```python
from build123d import *

# Parameters (mm, degrees)
F0_R     = 2.5
F1_DEPTH = 5
F2_R     = 15
F2_R_2   = 2.5
F3_DEPTH = 100
F4_SIZE2 = 99.99999
F4_SIZE  = 4.99999


# Not quite as in the source:
# - a fillet or chamfer is up to 0.001 mm smaller than in the source, because OpenCascade refuses the exact size


with BuildPart() as f1:
    # F0 (on Top) → F1 (new body)
    with BuildSketch(Plane.XY):
        with BuildLine():
            Line((7.4939975981, -22.8), (14.0512454964, -5.25))
            ThreePointArc((14.0512454964, -5.25), (0, 15), (-14.0512454964, -5.25))
            Line((-14.0512454964, -5.25), (-7.4939975981, -22.8))
            ThreePointArc((-7.4939975981, -22.8), (0, -28), (7.4939975981, -22.8))
        make_face()
        with Locations((0, -20)):
            Circle(F0_R, mode=Mode.SUBTRACT)
        Circle(F0_R, mode=Mode.SUBTRACT)
    extrude(amount=F1_DEPTH)

    # F2 (on face) → F3 (join)
    with BuildSketch(Plane.XY.offset(5)):
        Circle(F2_R)
        Circle(F2_R_2, mode=Mode.SUBTRACT)
    extrude(amount=F3_DEPTH)

    # F4 (size 5 and 100 in the source; OpenCascade refuses exactly that, so slightly less here)
    f4_edges = [f1.edges().sort_by_distance(p)[0] for p in [
        (-15, 0, 105),
    ]]
    f4_side = f1.faces().sort_by_distance((-14.575736, 0, 105))[0]
    chamfer(f4_edges, length=F4_SIZE, length2=F4_SIZE2, reference=f4_side)


solid = f1.part
```
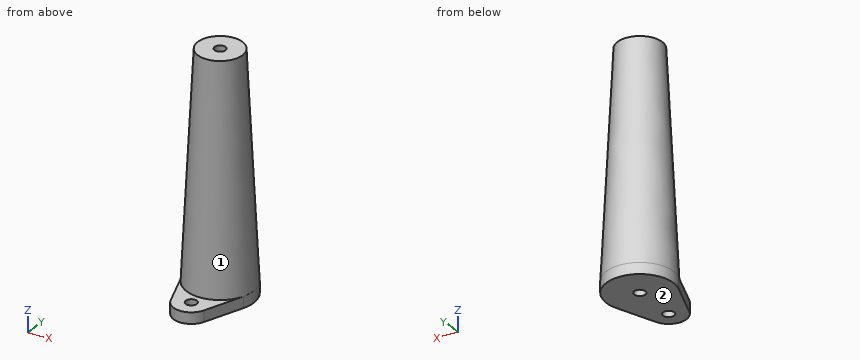
Verification items for the finished model (mm, model axes). Face numbers are marked on the shaded views. Coordinates: 2 decimals unless noted, no trailing zeros. Write each loop counter-clockwise with the first axis right and the second up, starting at its lowest first coordinate (ties: lowest second). Pieces come first, ordered by that corner, then holes. Notation, with made-up numbers: M 87,-3 L 131,-3 A16 cw 131,23 Z; hole C 62,-28 d4. An arc over 180 degrees is marked long. One line per item, written item: value.
Item 1: Scan lines: line 1 along Y through (x, z) = (0, 1.3); line 2 along Z through (x, y) = (4.5, -24.5); line 3 along Y through (x, z) = (0, 68). Record each from-to range of solid material in increasing order.
Check sheet entries:
line 1: y = -28 to -22.5, -17.5 to -2.5, 2.5 to 15
line 2: z = 0 to 5
line 3: y = -11.85 to -2.5, 2.5 to 11.85
Item 2: Gauge pin test, flat ends, axial feed: pin 1 Ø2 at (x, y) = (-7, 6.5) entering from -Z; pin 2 Ø3 at (x, z) = (-5.5, 85) entering from -Y; pin 3 Ø1 at (y, z) = (-6, 73) entering from -X; pin 4 Ø8 at (x, z) = (-6.5, 23.5) entering from +Y. Record the tip position at first contact, or that the pin passes through.
Check sheet entries:
pin 1: stops at z = 0
pin 2: stops at y = -10.25
pin 3: stops at x = -10.21
pin 4: stops at y = 13.88
Item 3: Mould release check, pull along Y, two halves, no side actions. Record for the marked faces 1 and 2: pulls with the +Y half, pulls with the -Y half, needs draft (parallel to the pull), parting line crosses it, or undercut.
Check sheet entries:
face 1: parting line crosses it
face 2: needs draft
Item 4: Section check A-A, the plane y = -20. Record the boundary of the cut face in (x, z).
Check sheet entries:
outline: M -8.54,0 L -2.5,0 L -2.5,5 L -8.54,5 Z; M 2.5,0 L 8.54,0 L 8.54,5 L 2.5,5 Z
Item 5: Section check B-B, the plane x = 0. State how many separate pieces and enclosed holes the cut face has, plus the area to 4 significant figures.
Check sheet entries:
separate pieces: 3
enclosed holes: 0
area: 2,165 mm^2
Item 6: Section check C-C, the plane z = 21. Record the boundary of the cut face in (x, y), plus the area to 3 significant figures.
Check sheet entries:
outline: C 0,0 d28.4; hole C 0,0 d5
area: 614 mm^2
Item 7: Section check D-D, the plane y = -24.5. Record the boundary of the cut face in (x, z), plus the area to 3 significant figures.
Check sheet entries:
outline: M -6.61,0 L 6.61,0 L 6.61,5 L -6.61,5 Z
area: 66.1 mm^2
